Study the drawing (mm; zero at the part's minimum x, y, z) and answer. A direction names the side the tool comes from. Coordinates: 2 decimals unless noted, no trailing zeros. Order: outer loops, then holes, each group sorted by start corner. A loop starts at its lowest first (then second) coordinate and runs counter-clockwise, first axis right, second up.
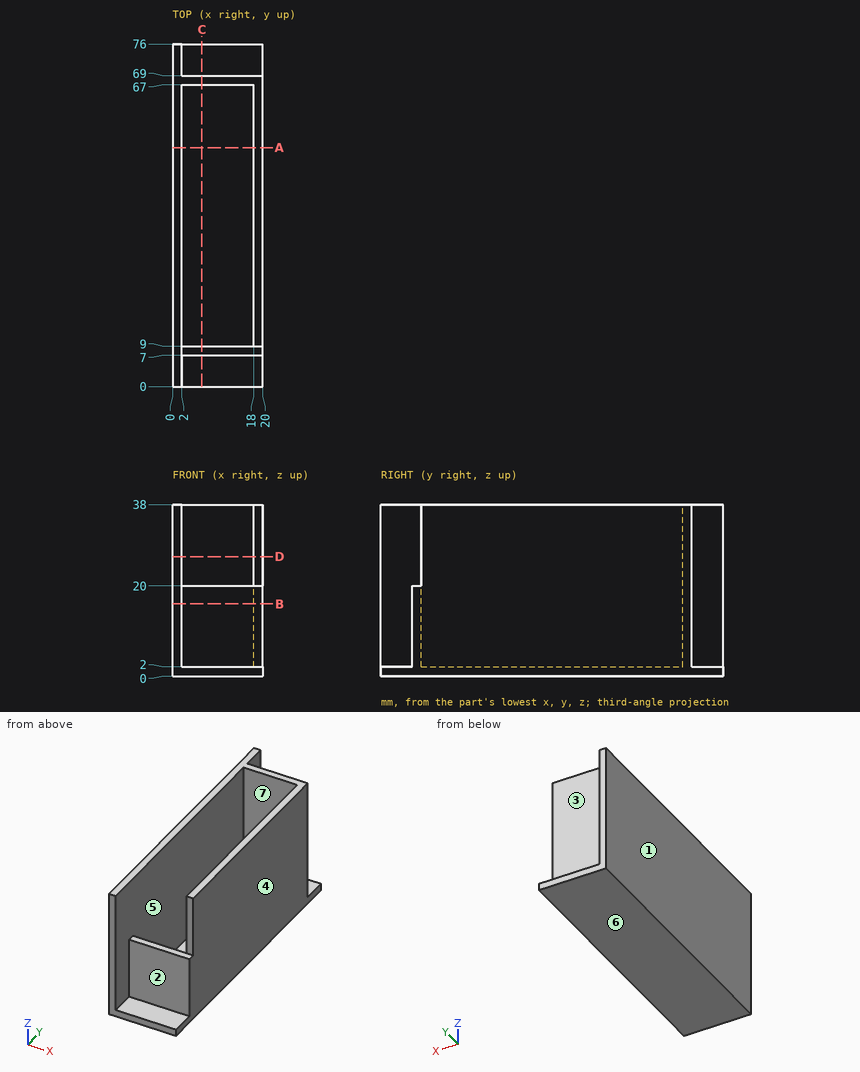
(1) Find section D-D (z = 26.5). Write down the section's boundary in (x, y).
(2) Find section C-C (x = 6.5). Write down the section's boundary in (y, z), and give its area (3 significant figures).
(3) Consider line 1 (X direction, y = 29.5, z = 28); line 2 (Y direction, x = 13.75, z = 8); line 3 (Z direction, x = 7.25, y = 12). Determine where each line is inside the solid, lowest interval first.
(4) The mould has two halves that part along X. Classify the marked faces 4, 5, 6 and 7: released by +X, released by -X, zero draft, split by the parting line, or undercut.
(5) Each of these flat-tipped pins is pushed along its axis until it touches: pin 1 Ø3 at (x, z) = (6, 22.5) entering from -Y; pin 2 Ø2 at (x, y) = (9, 8) entering from +Z; pin 3 Ø1.6 at (x, z) = (19.5, 28) entering from -Y. Where does it stop, or does it pass through?
(6) Find section B-B (z = 16). Write down the section's boundary in (x, y).
(7) For the marked faces 1, 2 and 3, determine the directions among +Z, -Z, +X, -X, +Y, -Y from which every point of the face is accessible in a straight line to the end or side of a thin tool.
(8) Find section A-A (y = 53). Write down the section's boundary in (x, z).
Findings below:
1. outline: (0, 0) - (2, 0) - (2, 67) - (18, 67) - (18, 9) - (20, 9) - (20, 69) - (2, 69) - (2, 76) - (0, 76) - close
2. outline: (0, 0) - (76, 0) - (76, 2) - (69, 2) - (69, 38) - (67, 38) - (67, 2) - (9, 2) - (9, 20) - (7, 20) - (7, 2) - (0, 2) - close
2. area: 260 mm2
3. line 1: x = 0 to 2, 18 to 20
3. line 2: y = 7 to 9, 67 to 69
3. line 3: z = 0 to 2
4. face 4: released by +X
4. face 5: undercut
4. face 6: zero draft
4. face 7: undercut
5. pin 1: stops at y = 67
5. pin 2: stops at z = 20
5. pin 3: stops at y = 9
6. outline: (0, 0) - (2, 0) - (2, 7) - (20, 7) - (20, 69) - (2, 69) - (2, 76) - (0, 76) - close; hole (2, 9) - (18, 9) - (18, 67) - (2, 67) - close
7. face 1: +Z, -Z, -X, +Y, -Y
7. face 2: +Z, +X, -Y
7. face 3: +Z, +X, +Y
8. outline: (0, 0) - (20, 0) - (20, 38) - (18, 38) - (18, 2) - (2, 2) - (2, 38) - (0, 38) - close
